Can you work these out from the drawing? Everything is in mm from the part's minimum corner. Give positions to 0.01 mm unless a question says otherwise; leave off trailing zeros. Order: outer loops, then holes, each group sorted by start corner. A loop starts at its lowest first (then second) coordinate and runs counter-clockwise, first axis right, second up. Notation, with made-up numbers: (89, -20.5) - (116, -20.5) arc R8 ccw to (116, -10.5) - close; hole circle Ø6 at (38, 31.5). An arc over 180 degrees is marked (long way). Answer as a JSON object with one key per item and string values.
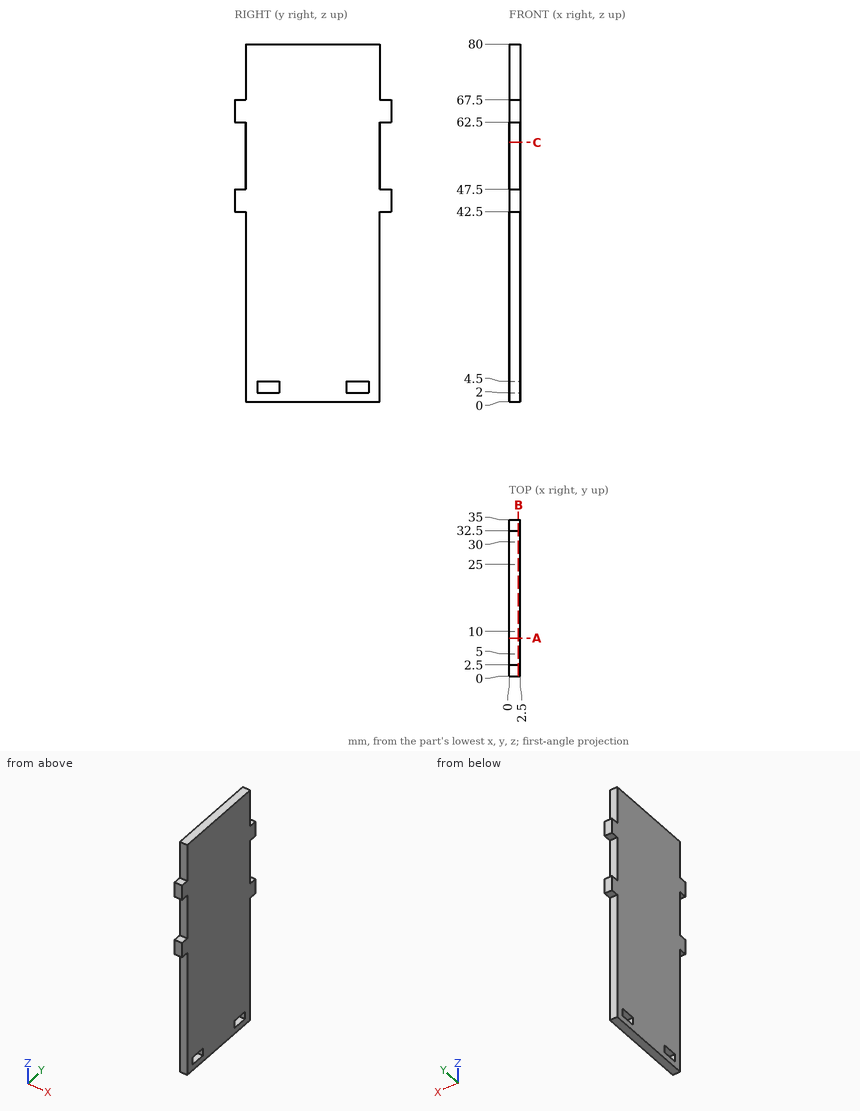
Q1. I need wall thicknesses on L1, parallel to Z at x = 1.95, y = 26; L2, parallel to Y at x = 2.1, z = 39. Which ranges of each line are inside material? Lowest first, please.
Recorded:
{"L1": "z = 0 to 2, 4.5 to 80", "L2": "y = 2.5 to 32.5"}
Q2. If we section it at A-A, the plane y = 8.5: Please give me the cut outline in (x, z), then the cut area to 3 significant figures.
Recorded:
{"outline": "(0, 0) - (2.5, 0) - (2.5, 2) - (0, 2) - close; (0, 4.5) - (2.5, 4.5) - (2.5, 80) - (0, 80) - close", "area": "194 mm^2"}
Q3. If we section it at B-B, the plane x = 2.05: Please give me the cut outline in (y, z), then the cut area to 4 significant figures.
Recorded:
{"outline": "(0, 42.5) - (2.5, 42.5) - (2.5, 0) - (32.5, 0) - (32.5, 42.5) - (35, 42.5) - (35, 47.5) - (32.5, 47.5) - (32.5, 62.5) - (35, 62.5) - (35, 67.5) - (32.5, 67.5) - (32.5, 80) - (2.5, 80) - (2.5, 67.5) - (0, 67.5) - (0, 62.5) - (2.5, 62.5) - (2.5, 47.5) - (0, 47.5) - close; hole (5, 2) - (10, 2) - (10, 4.5) - (5, 4.5) - close; hole (25, 2) - (30, 2) - (30, 4.5) - (25, 4.5) - close", "area": "2,425 mm^2"}
Q4. If we section it at C-C, the plane z = 58: Please give me the cut outline in (x, y).
Recorded:
{"outline": "(0, 2.5) - (2.5, 2.5) - (2.5, 32.5) - (0, 32.5) - close"}
Q5. I'm going to push a flat-ended pin straight in: pin 1 Ø0.8 at (x, z) = (1, 74) entering from +Y. Where does the tip first touch, or does it pass through?
Recorded:
{"pin 1": "stops at y = 32.5"}
